Part print with two shaded views. Sizes in mm from the minimum x, y, z corner. Round coordinates to 2 decimals unless told otherwise and drop trailing zeros. Order: outer loops, then holes, each group sorted by start corner. A loop starts at its lowest first (then second) coordinate and runs counter-clockwise, first axis right, second up. Notation, with made-up numbers: M 56.25,4 L 95.25,4 A12 cw 95.25,17 Z; hole C 24,47 d6. An arc over 180 degrees is marked long. Return JSON: item names as keys, results as strings. Group by question number.
Item 1: Slice it at A-A on y = 5. Write the cut outline in (x, z), then the cut area to 3 significant figures.
Item 2: Slice it at B-B on z = 25. Write the cut outline in (x, y).
Item 3: Pull direction Z, two halves, no side cores. Call the marked faces 1, 2 and 3: pulls with the +Z half, pulls with the -Z half, needs draft (parallel to the pull), parting line crosses it, or undercut.
Item 4: Pin check, flat tips, straight feed: pin 1 Ø3 at (y, z) = (5, 29) entering from +X; pin 2 Ø3 at (y, z) = (3.5, 10) entering from -X; pin 3 Ø13.5 at (x, z) = (23, 23.5) entering from +Y. Stop position of each tip, or through.
Item 5: Slice it at C-C on x = 25. Write the cut outline in (y, z).
Item 6: Slice it at D-D on y = 1.25. Write the cut outline in (x, z).
Item 7: Probe line 1 along Z through (x, y) = (25, 6.45); line 2 along Z through (x, y) = (25, 3.15). List the from-to ranges inside material, lowest first.
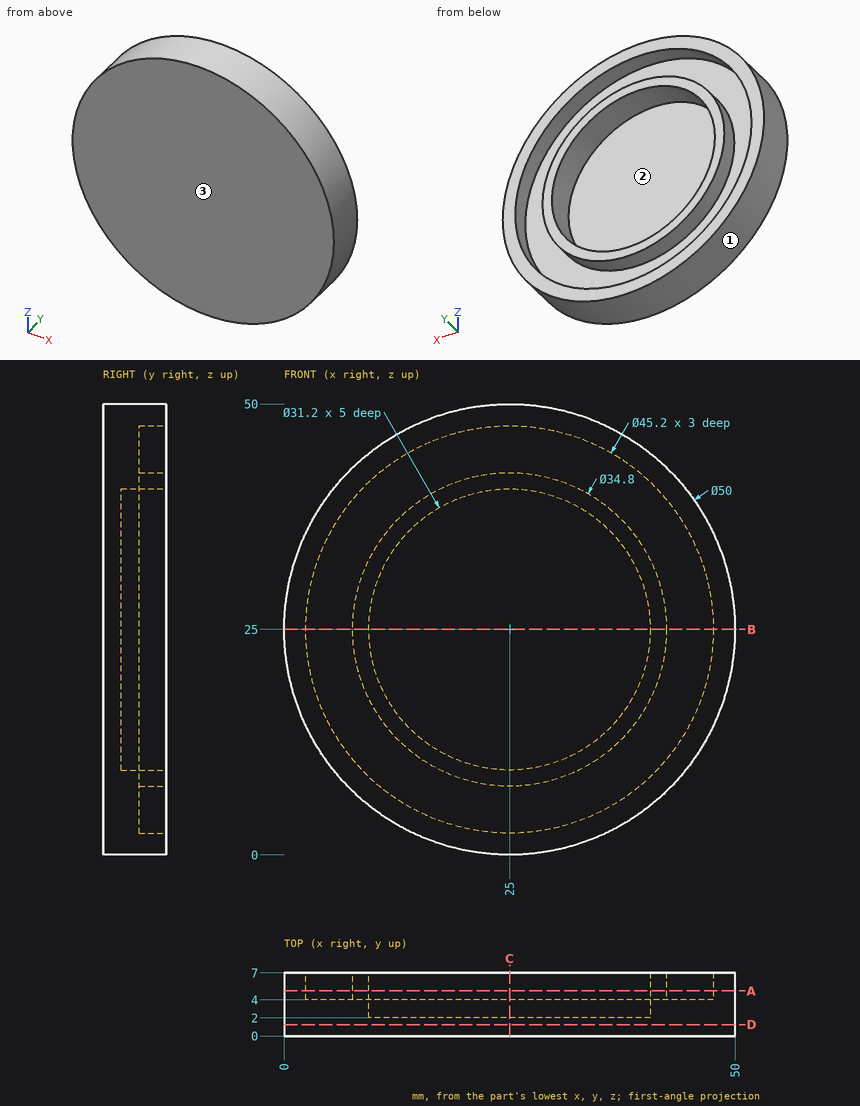
Output values:
{
 "1": {"outline": "C 25,25 d50; C 25,25 d34.8; hole C 25,25 d45.2; hole C 25,25 d31.2", "area": "546 mm²"},
 "2": {"outline": "M 0,0 L 50,0 L 50,7 L 47.6,7 L 47.6,4 L 42.4,4 L 42.4,7 L 40.6,7 L 40.6,2 L 9.4,2 L 9.4,7 L 7.6,7 L 7.6,4 L 2.4,4 L 2.4,7 L 0,7 Z"},
 "3": {"face 1": "parting line crosses it", "face 2": "undercut", "face 3": "needs draft"},
 "4": {"pin 1": "x = 49.87", "pin 2": "x = 3.96", "pin 3": "y = 2"},
 "5": {"outline": "M 0,0 L 7,0 L 7,2.4 L 4,2.4 L 4,7.6 L 7,7.6 L 7,9.4 L 2,9.4 L 2,40.6 L 7,40.6 L 7,42.4 L 4,42.4 L 4,47.6 L 7,47.6 L 7,50 L 0,50 Z"},
 "6": {"outline": "C 25,25 d50"},
 "7": {"line 1": "0 to 2.4, 7.6 to 9.4, 40.6 to 42.4, 47.6 to 50", "line 2": "0 to 9.4, 40.6 to 50"}
}
